Here's the drawing with two shaded views (mm, measured from the low corner). I have some questions. A direction names the side the tool comes from. Round coordinates to 2 decimals unless told otherwise and drop trailing zeros. Loops run counter-clockwise (first coordinate to the right, second up) from the corner with the lowest first, then second, coordinate; pieces in that order, holes last.
(1) I want a section at C-C on x = 4.5. Write out the boundary of the cut face in (y, z).
(2) Will these pins go through, and if not, where does the flat tip stop? pin 1 Ø2 at (y, z) = (13, 7.5) entering from -X; pin 2 Ø1 at (x, y) = (32.5, 15) entering from -Z; pin 3 Ø1 at (y, z) = (13, 1.5) entering from +X; pin 4 Ø1.8 at (x, z) = (4.5, 5.5) entering from +Y.
(3) Thinking about a two-plate mould opening in Z: for the marked faces 1, 2, 3 and 4, which applies, released by +Z, released by -Z, zero draft, split by the parting line, or undercut?
(4) Which directions (+Z, -Z, +X, -X, +Y, -Y) give clear straight access to the entire face, cutting with the end or side of a thin tool? Please do the marked faces 5 and 6.
(5) I want a section at D-D on z = 2. Write out the boundary of the cut face in (x, y) (1 decimal).
(6) I want a section at A-A on y = 11. Give the number of separate pieces and of enclosed holes in the cut face, plus the area to 3 significant figures.
(7) If I drill on line 1 along Z through (x, y) = (13.63, 19.2); line 2 along Y through (x, z) = (25, 8.5); line 3 along Y through (x, z) = (29, 9.75) (1 decimal), over which ranges is the centre line in solid material (lowest first)?
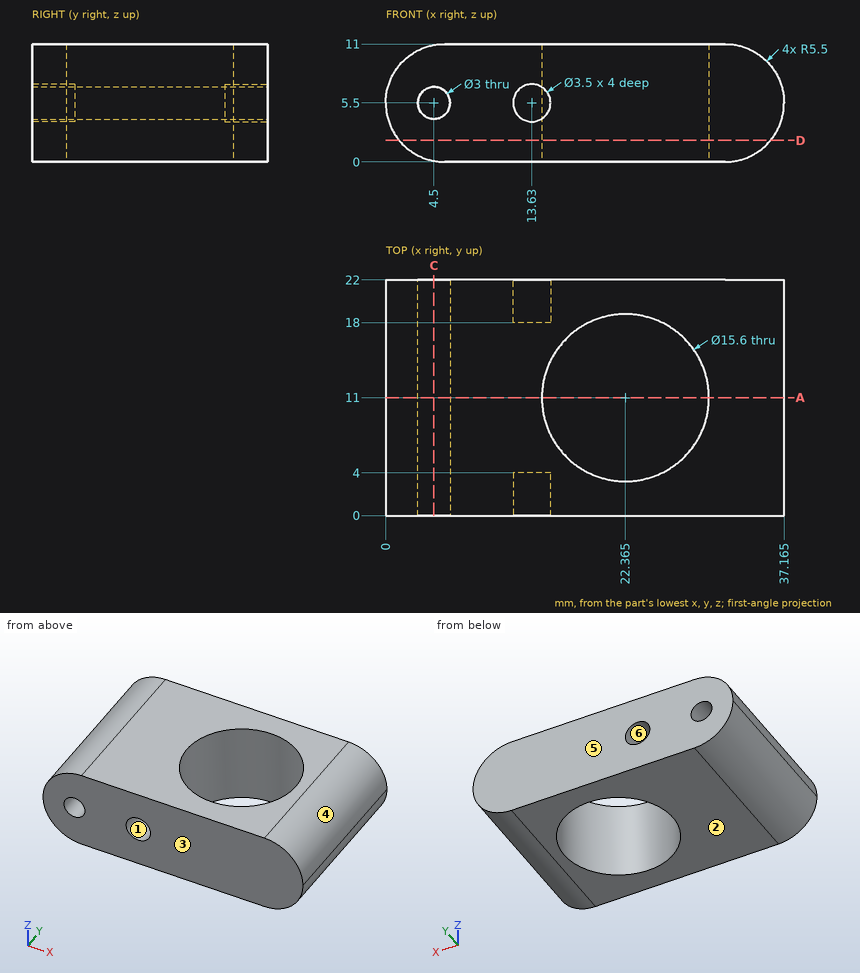
Filled sheet:
1. outline: (0, 0.09) - (22, 0.09) - (22, 4) - (0, 4) - close; (0, 7) - (22, 7) - (22, 10.91) - (0, 10.91) - close
2. pin 1: stops at x = 0.09
2. pin 2: stops at z = 0.01
2. pin 3: stops at x = 35.91
2. pin 4: passes through
3. face 1: undercut
3. face 2: released by -Z
3. face 3: zero draft
3. face 4: released by +Z
4. face 5: +Z, -Z, +X, -X, +Y
4. face 6: +Y
5. outline: (1.3, 0) - (35.9, 0) - (35.9, 22) - (1.3, 22) - close; hole circle Ø15.6 at (22.4, 11)
6. separate pieces: 2
6. enclosed holes: 1
6. area: 204 mm2
7. line 1: z = 0 to 3.75, 7.25 to 11
7. line 2: y = 0 to 3.66, 18.34 to 22
7. line 3: y = 0 to 6.9, 15.1 to 22
